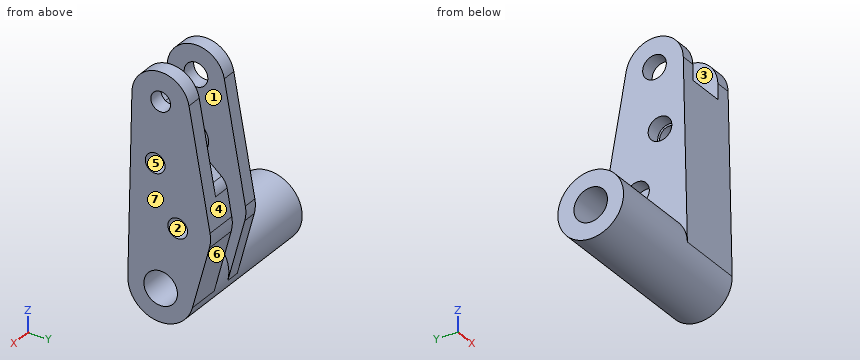
from build123d import *

# Parameters (mm, degrees)
BOSS_EXTRUDE1_DEPTH = 13.096874999999999
CUT_EXTRUDE4_START  = -6.35
CUT_EXTRUDE4_DEPTH  = 3.96875
CUT_EXTRUDE6_DEPTH  = 3.571875
SKETCH3_R           = 3.2385000000000006
SKETCH3_R_2         = 1.9049999999999998
SKETCH3_R_3         = 1.905
SKETCH3_R_4         = 1.9050000000000002
CUT_EXTRUDE2_DEPTH  = 44.62489589012807
SKETCH4_R           = 6.349999999999998
SKETCH4_R_2         = 3.2385000000000006
BOSS_EXTRUDE2_DEPTH = 18.653125
SKETCH5_R           = 2.286
SKETCH5_R_2         = 2.285999999999998
SKETCH5_R_3         = 2.2859999999999947
CUT_EXTRUDE5_DEPTH  = 2.778125
FILLET1_R           = 3.175


with BuildPart() as part:
    # Sketch1 → Boss-Extrude1 (new body)
    with BuildSketch(Plane(origin=(0, 0, 0), x_dir=(0, 0, -1), z_dir=(1, 0, 0))):
        with BuildLine():
            Line((-0.144318181818181, -6.348359808832252), (-35.051278409090905, -5.55481483272822))
            ThreePointArc((-35.051278409090905, -5.55481483272822), (-40.46435346310375, -0.4329864585648121), (-35.912861193635386, 5.467727528380438))
            Line((-35.912861193635386, 5.467727528380438), (-13.396242215168781, 9.535833333808146))
            ThreePointArc((-13.396242215168781, 9.535833333808146), (-12.00362991406523, 9.631527090305429), (-10.623757057470224, 9.420630869737527))
            Line((-10.623757057470224, 9.420630869737527), (1.643500936400966, 6.133628996935595))
            ThreePointArc((1.643500936400966, 6.133628996935595), (6.285849057186948, -0.9003341769931446), (-0.144318181818181, -6.348359808832252))
        make_face()
    extrude(amount=-BOSS_EXTRUDE1_DEPTH)

    # Sketch6 → Cut-Extrude4 (cut)
    with BuildSketch(Plane(origin=(0, 0, 0), x_dir=(0, 0, -1), z_dir=(1, 0, 0)).offset(CUT_EXTRUDE4_START)):
        with BuildLine():
            Line((1.643500936400966, 6.133628996935595), (-10.623757057470224, 9.420630869737526))
            ThreePointArc((-10.623757057470224, 9.420630869737526), (-12.00362991406523, 9.63152709030543), (-13.396242215168781, 9.535833333808146))
            Line((-13.396242215168781, 9.535833333808146), (-35.912861193635386, 5.467727528380437))
            ThreePointArc((-35.912861193635386, 5.467727528380437), (-40.46435346310375, -0.4329864585648108), (-35.051278409090905, -5.55481483272822))
            Line((-35.051278409090905, -5.55481483272822), (-31.977891932173424, -5.6246825720703155))
            ThreePointArc((-31.977891932173424, -5.6246825720703155), (-30.943788765977928, -4.9469644338822985), (-30.060617786194513, -4.081701321509548))
            Line((-30.060617786194513, -4.081701321509548), (-23.677913080624045, 3.524909941821936))
            Line((-23.677913080624045, 3.524909941821936), (-15.9094683647003, -1.9146136084331862))
            ThreePointArc((-15.9094683647003, -1.9146136084331862), (-10.095430083753156, -2.6800462691885727), (-6.133628996935595, 1.643500936400966))
            ThreePointArc((-6.133628996935595, 1.643500936400966), (-3.1750000000000385, 5.4992613140311635), (1.643500936400966, 6.133628996935595))
        make_face()
    extrude(amount=-CUT_EXTRUDE4_DEPTH, mode=Mode.SUBTRACT)

    # Sketch7 → Cut-Extrude6 (cut, symmetric)
    with BuildSketch(Plane(origin=(-6.5484374999999995, 0, 0), x_dir=(0, 0, -1), z_dir=(1, 0, 0))):
        with BuildLine():
            Line((-30.06061778619451, -4.0817013215095495), (-19.57011605971736, 8.420391799135219))
            Line((-19.57011605971736, 8.420391799135219), (-35.912861193635386, 5.467727528380437))
            ThreePointArc((-35.912861193635386, 5.467727528380437), (-40.46435346310375, -0.4329864585648108), (-35.051278409090905, -5.55481483272822))
            Line((-35.051278409090905, -5.55481483272822), (-31.977891932173424, -5.6246825720703155))
            ThreePointArc((-31.977891932173424, -5.6246825720703155), (-30.943788765977924, -4.946964433882303), (-30.06061778619451, -4.0817013215095495))
        make_face()
    extrude(amount=CUT_EXTRUDE6_DEPTH, both=True, mode=Mode.SUBTRACT)

    # Sketch3 → Cut-Extrude2 (cut, through all)
    with BuildSketch(Plane(origin=(0, 0, 0), x_dir=(0, 0, -1), z_dir=(1, 0, 0))):
        Circle(SKETCH3_R)
        with Locations((-34.925, 0)):
            Circle(SKETCH3_R_2)
        with Locations((-12.26725799387119, 3.287001872801932)):
            Circle(SKETCH3_R_3)
        with Locations((-23.07385471451217, -1.0633688768983705)):
            Circle(SKETCH3_R_4)
    extrude(amount=-CUT_EXTRUDE2_DEPTH, mode=Mode.SUBTRACT)

    # Sketch4 → Boss-Extrude2 (add)
    with BuildSketch(Plane.ZY.offset(13.096874999999999)):
        with Locations(Location((0, 0, 0), (0, 0, 180))):
            Circle(SKETCH4_R)
        with Locations(Location((0, 0, 0), (0, 0, 180))):
            Circle(SKETCH4_R_2, mode=Mode.SUBTRACT)
    extrude(amount=BOSS_EXTRUDE2_DEPTH)

    # Sketch5 → Cut-Extrude5 (cut)
    with BuildSketch(Plane.ZY.offset(13.096874999999999)):
        with Locations((12.26725799387119, 3.287001872801932)):
            Circle(SKETCH5_R)
        with Locations((23.07385471451217, -1.0633688768983705)):
            Circle(SKETCH5_R_2)
        with Locations((34.925, 0)):
            Circle(SKETCH5_R_3)
    extrude(amount=-CUT_EXTRUDE5_DEPTH, mode=Mode.SUBTRACT)

    # Fillet1
    fillet1_edges = [part.edges().sort_by_distance(p)[0] for p in [
        (-8.334375, 3.524909941821936, 23.677913080624045),
        (-4.66328125, 8.420391799135219, 19.57011605971736),
    ]]
    fillet(fillet1_edges, radius=FILLET1_R)


solid = part.part
Design review of the part built by this model. Coordinates are the model's own, in mm. Face numbers are marked on the shaded views. A direction names the side the tool comes from. Round coordinates to 2 decimals unless told otherwise and drop trailing zeros. Write each loop counter-clockwise with the first axis right and the second up, starting at its lowest first coordinate (ties: lowest second). Pieces come first, ordered by that corner, then holes. Notation, with made-up numbers: (52.25, -17) -> (104.25, -17) arc R23 cw to (104.25, -9) -> close; hole circle Ø11 at (-10.75, 7.5). An arc over 180 degrees is marked (long way). One line per item, written item: value. Start each with the question number.
Q1. The part is to be moulded in two halves that separate along Z. For the marked faces 4, 5, 6 and 7, say which applies: pulls with the +Z half, pulls with the -Z half, needs draft (parallel to the pull), parting line crosses it, or undercut.
Q2. Add section C-C (z = 9). Give the boundary of the cut face in (x, y), then the cut area to 3 significant figures.
Q3. To check wall thickness, follow probe 1 along X at (y, z) = (5.5, 16.5); probe 2 along X at (y, z) = (-5.25, 5.5); probe 3 along Z at (x, y) = (-25.5, 0.25). State the ranges of each line that lie inside material, in increasing order.
Q4. Add section B-B (x = -15.5). Give the boundary of the cut face in (y, z).
Q5. Tool access review of the marked faces 1, 2 and 3: name each direction out of +Z, -Z, +X, -X, +Y, -Y from which nothing blocks a thin tool from reaching the whole face with its end or side.
Q6. Insertion check: P1, Ø1, axis at x = -4.5, z = 25, coming from the -Y side; P2, Ø1.5, axis at x = -16.5, z = 6.5, coming from the +Y side; P3, Ø3, axis at y = -1.06, z = 23.07, coming from the -X side; P4, Ø5, axis at y = -2, z = 24, coming from the -X side. Each pin has a flat end and moves straight along its axis. Give the tip position at first contact, or say it passes through.
Response:
1. face 4: pulls with the +Z half
1. face 5: undercut
1. face 6: pulls with the -Z half
1. face 7: needs draft
2. outline: (-13.1, -6.15) -> (0, -6.15) -> (0, 8.99) -> (-6.35, 8.99) -> (-6.35, -2.16) -> (-10.32, -2.16) -> (-10.32, 8.99) -> (-13.1, 8.99) -> close
2. area: 154 mm^2
3. probe 1: x = -13.1 to -10.32, -6.35 to 0
3. probe 2: x = -13.1 to 0
3. probe 3: z = -6.35 to -3.23, 3.23 to 6.35
4. outline: circle Ø12.7 at (0, 0); hole circle Ø6.48 at (0, 0)
5. face 1: +Y
5. face 2: +X, -X
5. face 3: +Z, +Y
6. P1: stops at y = -5.79
6. P2: stops at y = 2.69
6. P3: passes through
6. P4: stops at x = -13.1
